from build123d import *

# Parameters (mm, degrees)
F0_R     = 6
F1_DEPTH = 0.5
F3_DEPTH = 1
F4_R     = 0.6
F5_DEPTH = 25
F7_DEPTH = 0.4


with BuildPart() as f1:
    # F0 (on Top) → F1 (new body)
    with BuildSketch(Plane.XY):
        Polygon((3.6084391824, 6.25), (0, 12.5), (-3.6084391824, 6.25), align=None)
        Polygon((2, 6.7328579847), (-2, 6.7328579847), (0, 10.1969595999), align=None, mode=Mode.SUBTRACT)
        Polygon((3.6084391824, 6.25), (-3.6084391824, 6.25), (-7.2168783649, 0), (-3.6084391824, -6.25), (3.6084391824, -6.25), (7.2168783649, 0), align=None)
        Circle(F0_R, mode=Mode.SUBTRACT)
        Polygon((-7.2168783649, 0), (-3.6084391824, 6.25), (-10.8253175473, 6.25), align=None)
        Polygon((-8.8308260548, 5.0984797999), (-4.8308260548, 5.0984797999), (-6.8308260548, 1.6343781848), align=None, mode=Mode.SUBTRACT)
        Polygon((10.8253175473, 6.25), (3.6084391824, 6.25), (7.2168783649, 0), align=None)
        Polygon((8.8308260548, 5.0984797999), (6.8308260548, 1.6343781848), (4.8308260548, 5.0984797999), align=None, mode=Mode.SUBTRACT)
        Polygon((-3.6084391824, -6.25), (-7.2168783649, 0), (-10.8253175473, -6.25), align=None)
        Polygon((-8.8308260548, -5.0984797999), (-6.8308260548, -1.6343781848), (-4.8308260548, -5.0984797999), align=None, mode=Mode.SUBTRACT)
        Polygon((10.8253175473, -6.25), (7.2168783649, 0), (3.6084391824, -6.25), align=None)
        Polygon((8.8308260548, -5.0984797999), (4.8308260548, -5.0984797999), (6.8308260548, -1.6343781848), align=None, mode=Mode.SUBTRACT)
        Polygon((3.6084391824, -6.25), (-3.6084391824, -6.25), (0, -12.5), align=None)
        Polygon((0, -10.1969595999), (-2, -6.7328579847), (2, -6.7328579847), align=None, mode=Mode.SUBTRACT)
    extrude(amount=F1_DEPTH)

    # F2 (on Top) → F3 (join)
    with BuildSketch(Plane.XY):
        with BuildLine():
            Line((0, 9.2784009988), (-1.7186464041, 4.6953439211))
            ThreePointArc((-1.7186464041, 4.6953439211), (-2.5, 4.3301270189), (-3.2069639131, 3.8360634066))
            Line((-3.2069639131, 3.8360634066), (-8.0353309714, 4.6392004994))
            Line((-8.0353309714, 4.6392004994), (-4.9256103173, 0.8592805145))
            ThreePointArc((-4.9256103173, 0.8592805145), (-5, 0), (-4.9256103173, -0.8592805145))
            Line((-4.9256103173, -0.8592805145), (-8.0353309714, -4.6392004994))
            Line((-8.0353309714, -4.6392004994), (-3.2069639131, -3.8360634066))
            ThreePointArc((-3.2069639131, -3.8360634066), (-2.5, -4.3301270189), (-1.7186464041, -4.6953439211))
            Line((-1.7186464041, -4.6953439211), (0, -9.2784009988))
            Line((0, -9.2784009988), (1.7186464041, -4.6953439211))
            ThreePointArc((1.7186464041, -4.6953439211), (2.5, -4.3301270189), (3.2069639131, -3.8360634066))
            Line((3.2069639131, -3.8360634066), (8.0353309714, -4.6392004994))
            Line((8.0353309714, -4.6392004994), (4.9256103173, -0.8592805145))
            ThreePointArc((4.9256103173, -0.8592805145), (5, 0), (4.9256103173, 0.8592805145))
            Line((4.9256103173, 0.8592805145), (8.0353309714, 4.6392004994))
            Line((8.0353309714, 4.6392004994), (3.2069639131, 3.8360634066))
            ThreePointArc((3.2069639131, 3.8360634066), (2.5, 4.3301270189), (1.7186464041, 4.6953439211))
            Line((1.7186464041, 4.6953439211), (0, 9.2784009988))
        make_face()
        Polygon((-4.7051270189, -1.8504809472), (-3.9551270189, -3.1495190528), (-6.0621778265, -3.5), align=None, mode=Mode.SUBTRACT)
        Polygon((-0.75, -5), (0.75, -5), (0, -7), align=None, mode=Mode.SUBTRACT)
        Polygon((3.9551270189, -3.1495190528), (4.7051270189, -1.8504809472), (6.0621778265, -3.5), align=None, mode=Mode.SUBTRACT)
        Polygon((-3.9551270189, 3.1495190528), (-4.7051270189, 1.8504809472), (-6.0621778265, 3.5), align=None, mode=Mode.SUBTRACT)
        Polygon((4.7051270189, 1.8504809472), (3.9551270189, 3.1495190528), (6.0621778265, 3.5), align=None, mode=Mode.SUBTRACT)
        Polygon((-0.75, 5), (0, 7), (0.75, 5), align=None, mode=Mode.SUBTRACT)
        with BuildLine():
            ThreePointArc((-3.2069639131, 3.8360634066), (-2.5, 4.3301270189), (-1.7186464041, 4.6953439211))
            Line((-1.7186464041, 4.6953439211), (-5, 8.6602540378))
            Line((-5, 8.6602540378), (-3.2069639131, 3.8360634066))
        make_face()
        with BuildLine():
            Line((5, 8.6602540378), (1.7186464041, 4.6953439211))
            ThreePointArc((1.7186464041, 4.6953439211), (2.5, 4.3301270189), (3.2069639131, 3.8360634066))
            Line((3.2069639131, 3.8360634066), (5, 8.6602540378))
        make_face()
        with BuildLine():
            ThreePointArc((-4.9256103173, -0.8592805145), (-5, 0), (-4.9256103173, 0.8592805145))
            Line((-4.9256103173, 0.8592805145), (-10, 0))
            Line((-10, 0), (-4.9256103173, -0.8592805145))
        make_face()
        with BuildLine():
            Line((10, 0), (4.9256103173, 0.8592805145))
            ThreePointArc((4.9256103173, 0.8592805145), (5, 0), (4.9256103173, -0.8592805145))
            Line((4.9256103173, -0.8592805145), (10, 0))
        make_face()
        with BuildLine():
            ThreePointArc((-1.7186464041, -4.6953439211), (-2.5, -4.3301270189), (-3.2069639131, -3.8360634066))
            Line((-3.2069639131, -3.8360634066), (-5, -8.6602540378))
            Line((-5, -8.6602540378), (-1.7186464041, -4.6953439211))
        make_face()
        with BuildLine():
            Line((5, -8.6602540378), (3.2069639131, -3.8360634066))
            ThreePointArc((3.2069639131, -3.8360634066), (2.5, -4.3301270189), (1.7186464041, -4.6953439211))
            Line((1.7186464041, -4.6953439211), (5, -8.6602540378))
        make_face()
    extrude(amount=F3_DEPTH)

    # F4 (on face) → F5 (cut)
    with BuildSketch(Plane.XY.offset(1)):
        Polygon((0.75, 5), (-0.75, 5), (0, 3.4), align=None)
        Polygon((2.3652717414, 4.0967708298), (0.692820323, 3), (0.692820323, 1.2), (2.2516660498, 2.1), align=None)
        Polygon((-2.9444863729, 1.7), (-3.9551270189, 3.1495190528), (-4.7051270189, 1.8504809472), align=None)
        Polygon((-0.692820323, 3), (-2.3652717414, 4.0967708298), (-2.2516660498, 2.1), (-0.692820323, 1.2), align=None)
        Polygon((-2.9444863729, -1.7), (-4.7051270189, -1.8504809472), (-3.9551270189, -3.1495190528), align=None)
        Polygon((-2.9444863729, 0.9), (-4.7305434828, 0), (-2.9444863729, -0.9), (-1.3856406461, 0), align=None)
        Polygon((0, -3.4), (-0.75, -5), (0.75, -5), align=None)
        Polygon((-2.2516660498, -2.1), (-2.3652717414, -4.0967708298), (-0.692820323, -3), (-0.692820323, -1.2), align=None)
        Polygon((2.9444863729, -1.7), (3.9551270189, -3.1495190528), (4.7051270189, -1.8504809472), align=None)
        Polygon((0.692820323, -3), (2.3652717414, -4.0967708298), (2.2516660498, -2.1), (0.692820323, -1.2), align=None)
        Polygon((2.9444863729, 1.7), (4.7051270189, 1.8504809472), (3.9551270189, 3.1495190528), align=None)
        Polygon((2.9444863729, -0.9), (4.7305434828, 0), (2.9444863729, 0.9), (1.3856406461, 0), align=None)
        Circle(F4_R)
    extrude(amount=-F5_DEPTH, mode=Mode.SUBTRACT)

    # F6 (on face) → F7 (cut)
    with BuildSketch(Plane.XY.offset(1)):
        Polygon((0, 2.5456578814), (-0.692820323, 3), (-0.692820323, 1.2), (-2.2516660498, 2.1), (-2.2046043947, 1.2728289407), (-2.9444863729, 0.9), (-1.3856406461, 0), (-2.9444863729, -0.9), (-2.2046043947, -1.2728289407), (-2.2516660498, -2.1), (-0.692820323, -1.2), (-0.692820323, -3), (0, -2.5456578814), (0.692820323, -3), (0.692820323, -1.2), (2.2516660498, -2.1), (2.2046043947, -1.2728289407), (2.9444863729, -0.9), (1.3856406461, 0), (2.9444863729, 0.9), (2.2046043947, 1.2728289407), (2.2516660498, 2.1), (0.692820323, 1.2), (0.692820323, 3), align=None)
    extrude(amount=-F7_DEPTH, mode=Mode.SUBTRACT)


solid = f1.part
Geometry check sheet. Reference: the model listing, model coordinates, mm. A direction names the side the tool comes from. Round coordinates to 2 decimals unless told otherwise and drop trailing zeros. Loops run counter-clockwise (first coordinate to the right, second up) from the corner with the lowest first, then second, coordinate; pieces in that order, holes last.
Item 1: Cross-section at A-A on x = 8.5. Record the boundary of the cut face in (y, z).
Item 2: Gauge pin test, flat ends, axial feed: pin 1 (3 mm diameter, centred on x = 8, y = 4.5, fed in from +Z); pin 2 (0.6 mm diameter, centred on x = 6, z = 0.5, fed in from -Y). Record the tip position at first contact, or that the pin passes through.
Item 3: Thickness scan on line 1 (X direction, y = 0.5, z = 0.3); line 2 (X direction, y = -8, z = 0.4); line 3 (X direction, y = -7.5, z = 0.2). Record the ranges inside material, lowest first.
Item 4: Cross-section at B-B on y = 7.5. Record the boundary of the cut face in (x, z), then the cut area to 3 significant figures.
Item 5: Cross-section at C-C on z = 0.8. Count the separate pieces of the cut face and the enclosed holes in it, then the cut area to 3 significant figures.
Item 6: Access from +Z, -Z, +X, -X, +Y, -Y to the whole of each face (thin tool, end or side, straight path). Record for faces 1 (the flat face through (2.15, -0.44, 0.3)), 2 (the flat face through (9.12, 3.3, 0.25)), 3 (the flat face through (-9.12, -3.3, 0.25)).
Answer sheet:
1. outline: (-6.25, 0) - (-5.1, 0) - (-5.1, 0.5) - (-6.25, 0.5) - close; (-4.53, 0) - (-2.22, 0) - (-2.22, 0.5) - (-4.53, 0.5) - close; (-0.25, 0) - (0.25, 0) - (0.25, 1) - (-0.25, 1) - close; (2.22, 0) - (4.53, 0) - (4.53, 0.5) - (2.22, 0.5) - close; (5.1, 0) - (6.25, 0) - (6.25, 0.5) - (5.1, 0.5) - close
2. pin 1: stops at z = 1
2. pin 2: stops at y = -6.25
3. line 1: x = -7.51 to -3.74, -2.25 to -0.33, 0.33 to 2.25, 3.74 to 7.51
3. line 2: x = -4.75 to -4.45, -2.6 to -1.27, -0.48 to 0.48, 1.27 to 2.6, 4.45 to 4.75
3. line 3: x = -4.57 to -4.04, -2.89 to -1.56, -0.67 to 0.67, 1.56 to 2.89, 4.04 to 4.57
4. outline: (-4.57, 0) - (-4.04, 0) - (-4.04, 1) - (-4.57, 1) - close; (-2.89, 0) - (-1.56, 0) - (-1.56, 0.5) - (-2.89, 0.5) - close; (-0.67, 0) - (0.67, 0) - (0.67, 1) - (-0.67, 1) - close; (1.56, 0) - (2.89, 0) - (2.89, 0.5) - (1.56, 0.5) - close; (4.04, 0) - (4.57, 0) - (4.57, 1) - (4.04, 1) - close
4. area: 3.72 mm2
5. separate pieces: 1
5. enclosed holes: 7
5. area: 94.9 mm2
6. face 1: +Z, -Z
6. face 2: +Z, -Z, +X
6. face 3: +Z, -Z, -X
